```python
from build123d import *

# Parameters (mm, degrees)
SKETCH1_W           = 164
SKETCH1_H           = 54
BOSS_EXTRUDE1_DEPTH = 9.5
SKETCH3_W           = 49
SKETCH3_H           = 25.6
BOSS_EXTRUDE2_DEPTH = 8
SKETCH5_W           = 80
SKETCH5_H           = 36
BOSS_EXTRUDE3_DEPTH = 8.6


with BuildPart() as part:
    # Sketch1 → Boss-Extrude1 (new body)
    with BuildSketch(Plane(origin=(0, 0, 0), x_dir=(1, 0, 0), z_dir=(0, 1, 0))):
        with Locations((82, 27)):
            Rectangle(SKETCH1_W, SKETCH1_H)
    extrude(amount=BOSS_EXTRUDE1_DEPTH)

    # Sketch3 → Boss-Extrude2 (add)
    with BuildSketch(Plane(origin=(0, 9.5, 0), x_dir=(1, 0, 0), z_dir=(0, 1, 0))):
        with Locations((24.5, 27)):
            Rectangle(SKETCH3_W, SKETCH3_H)
    extrude(amount=BOSS_EXTRUDE2_DEPTH)

    # Sketch5 → Boss-Extrude3 (add)
    with BuildSketch(Plane(origin=(0, 9.5, 0), x_dir=(1, 0, 0), z_dir=(0, 1, 0))):
        with Locations((124, 20)):
            Rectangle(SKETCH5_W, SKETCH5_H)
    extrude(amount=BOSS_EXTRUDE3_DEPTH)


solid = part.part
```
Check sheet for the modelled part. Datum: model origin and axes. Units: mm. A direction names the side the tool comes from. Round coordinates to 2 decimals unless told otherwise and drop trailing zeros. Loops run counter-clockwise (first coordinate to the right, second up) from the corner with the lowest first, then second, coordinate; pieces in that order, holes last. Notation, with made-up numbers: M 30,43.25 L 69,43.25 A18 ccw 69,78.25 Z; hole C 57,43 d3. An arc over 180 degrees is marked long. Answer as a JSON object with one key per item and string values.
1. Mould release check, pull along X, two halves, no side actions. Record for faces 1 (the flat face through (123, 18.1, -20)), 2 (the flat face through (49, 13, -27)), 3 (the flat face through (0, 7, -27)): pulls with the +X half, pulls with the -X half, needs draft (parallel to the pull), parting line crosses it, or undercut.
Reply:
{"face 1": "needs draft", "face 2": "undercut", "face 3": "pulls with the -X half"}
2. Section check A-A (y = 16). Record the boundary of the cut face in (x, z).
Reply:
{"outline": "M 0,-39.8 L 49,-39.8 L 49,-14.2 L 0,-14.2 Z; M 84,-38 L 164,-38 L 164,-2 L 84,-2 Z"}
3. Section check C-C (z = -21). Record the boundary of the cut face in (x, y), plus the area to 3 significant figures.
Reply:
{"outline": "M 0,0 L 164,0 L 164,18.1 L 84,18.1 L 84,9.5 L 49,9.5 L 49,17.5 L 0,17.5 Z", "area": "2,640 mm²"}
4. Scan lines: line 1 (X direction, y = 15.5, z = -18); line 2 (Y direction, x = 126, z = -49.5); line 3 (X direction, y = 10.5, z = -14). Record each from-to range of solid material in increasing order.
Reply:
{"line 1": "x = 0 to 49, 84 to 164", "line 2": "y = 0 to 9.5", "line 3": "x = 84 to 164"}
5. Section check D-D (z = -48). Record the boundary of the cut face in (x, y).
Reply:
{"outline": "M 0,0 L 164,0 L 164,9.5 L 0,9.5 Z"}
6. Section check B-B (x = 122). Record the boundary of the cut face in (y, z), plus the area to 3 significant figures.
Reply:
{"outline": "M 0,-54 L 9.5,-54 L 9.5,-38 L 18.1,-38 L 18.1,-2 L 9.5,-2 L 9.5,0 L 0,0 Z", "area": "823 mm²"}
7. Gauge pin test, flat ends, axial feed: P1, Ø9.5, axis at x = 138, y = 14.5, coming from the -Z side; P2, Ø4.5, axis at x = 116.5, y = 14.5, coming from the +Z side; P3, Ø6, axis at x = 87.5, z = -42, coming from the +Y side. Record the tip position at first contact, or that the pin passes through.
Reply:
{"P1": "stops at z = -38", "P2": "stops at z = -2", "P3": "stops at y = 9.5"}
8. Access from +Z, -Z, +X, -X, +Y, -Y to the whole of each face (thin tool, end or side, straight path). Record for faces 4 (the flat face through (84, 14, -20)), 5 (the flat face through (24, 13, -39.8)), 6 (the flat face through (123, 14, -38)), 7 (the flat face through (123, 14, -2)).
Reply:
{"face 4": "+Z, -Z, +Y", "face 5": "-Z, +X, -X, +Y", "face 6": "-Z, +X, +Y", "face 7": "+Z, +X, -X, +Y"}
